Part print with two shaded views. Sizes in mm from the minimum x, y, z corner. A direction names the side the tool comes from. Coordinates: 2 decimals unless noted, no trailing zeros. Write each loop counter-clockwise with the first axis right and the second up, starting at its lowest first coordinate (ties: lowest second). Pieces come first, ordered by that corner, then holes. Notation, with made-up numbers: (-15, 41) - (10, 41) arc R25 cw to (10, 56) - close; hole circle Ø1 at (-31.75, 84). An arc over 180 degrees is marked (long way). One line per question, with ' | ' between items. Start each with the question number.
1. Which spindle directions (+Z, -Z, +X, -X, +Y, -Y) get a long thin tool onto all of the face, cutting with end or side? Do the marked faces 1, 2, 3 and 4. Say none if no direction does.
2. Band-saw the part on D-D, the plane x = 70. Write the cut outline in (y, z).
3. Band-saw the part on A-A, the plane z = 7. Write the cut outline in (x, y), then the cut area to 3 significant figures.
4. Band-saw the part on C-C, the plane x = 36. Write the cut outline in (y, z).
5. Probe line 1 (Y direction, x = 77.5, z = 15); line 2 (X direction, y = 30, z = 31); line 3 (Z direction, x = 19.5, y = 8). List the from-to ranges inside material, lowest first.
6. Band-saw the part on B-B, the plane y = 59.5. Write the cut outline in (x, z), then the cut area to 3 significant figures.
7. Flat gauge pins, fed straight in: P1, Ø14.5, axis at y = 23, z = 51, coming from the +X side; P2, Ø1.5, axis at x = 76.5, y = 53.5, coming from the +Z side (1 decimal); P3, Ø4, axis at x = 19, y = 52.5, coming from the +Z side. Where does each tip first touch, or does it go through?
8. Two-plate mould, pull along X, no slides. Class the marked faces 5, 6 and 7: +X half, -X half, draft (parallel to the pull), parting line (faces both ways), or undercut.
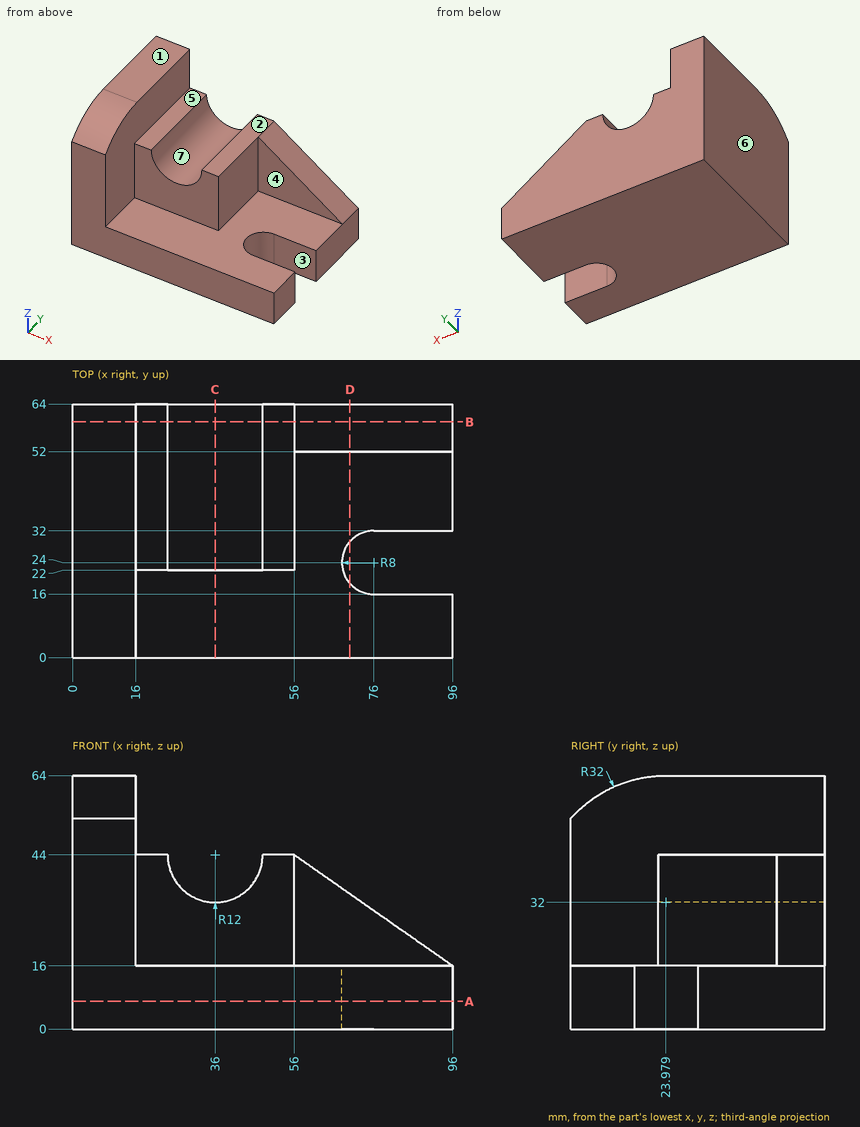
Filled in:
1) face 1: +Z, +X, -X, +Y, -Y | face 2: +Z, +X, +Y, -Y | face 3: +Z, -Z, +X | face 4: +Z, +X, -Y
2) outline: (0, 0) - (18.71, 0) - (18.71, 16) - (0, 16) - close; (29.29, 0) - (64, 0) - (64, 34.2) - (52, 34.2) - (52, 16) - (29.29, 16) - close
3) outline: (0, 0) - (96, 0) - (96, 16) - (76, 16) arc R8 cw to (76, 32) - (96, 32) - (96, 64) - (0, 64) - close | area: 5,720 mm²
4) outline: (0, 0) - (64, 0) - (64, 32) - (22, 32) - (22, 16) - (0, 16) - close
5) line 1: y = 0 to 16, 32 to 64 | line 2: x = 0 to 56 | line 3: z = 0 to 16
6) outline: (0, 0) - (96, 0) - (96, 16) - (56, 44) - (48, 44) arc R12 cw to (24, 44) - (16, 44) - (16, 64) - (0, 64) - close | area: 3,760 mm²
7) P1: stops at x = 56 | P2: stops at z = 30.2 | P3: stops at z = 44
8) face 5: draft | face 6: -X half | face 7: undercut
